Design review of the part shown in the three views and the two pictorial views. Dimensions are in mm from the part's minimum x, y and z. A direction names the side the tool comes from. Round coordinates to 2 decimals unless told otherwise and drop trailing zeros. Loops run counter-clockwise (first coordinate to the right, second up) from the corner with the lowest first, then second, coordinate; pieces in that order, holes last. Notation, with made-up numbers: M 6.25,13 L 61.25,13 A33 ccw 61.25,47 Z; hole C 62.25,75.5 d4. An arc over 180 degrees is marked long. Return JSON: item names as keys, results as strings. Group by question number.
Q1. Consider section C-C (z = 68). State the section outline as (x, y) points.
Q2. Clearance check with flat-ended pins moving along their axes: pin 1 Ø4 at (y, z) = (99, 36) entering from +X; pin 2 Ø11 at (x, z) = (128, 73.5) entering from +Y; pin 3 Ø1 at (x, z) = (59.5, 34.5) entering from +Y. State where each tip first meets the part, or that it passes through.
Q3. Consider section B-B (x = 67.5). State the section outline as (y, z) points, and give its area (3 significant figures).
Q4. For the marked faces 4, 5, 6 and 7, list the 3-axis set-ups (+Z, -Z, +X, -X, +Y, -Y) from which the entire face can be reached by the end or side of a thin tool; tool diameter is ignored.
Q5. Draft analysis for pull direction X (two halves, no side actions). For the marked faces 1, 2 and 3, state which applies: pulls with the +X half, pulls with the -X half, needs draft (parallel to the pull), parting line crosses it, or undercut.
Q6. Consider section A-A (y = 55). State the section outline as (x, z) points.
Q7. To check wall thickness, follow line 1 along X through (y, z) = (70.5, 10.5); line 2 along X through (y, z) = (42, 4.5); line 3 along Y through (x, z) = (14.5, 66.5). State the ranges of each line that lie inside material, in increasing order.
Q8. Consider section D-D (y = 97). State the section outline as (x, z) points, and give its area (3 significant figures).
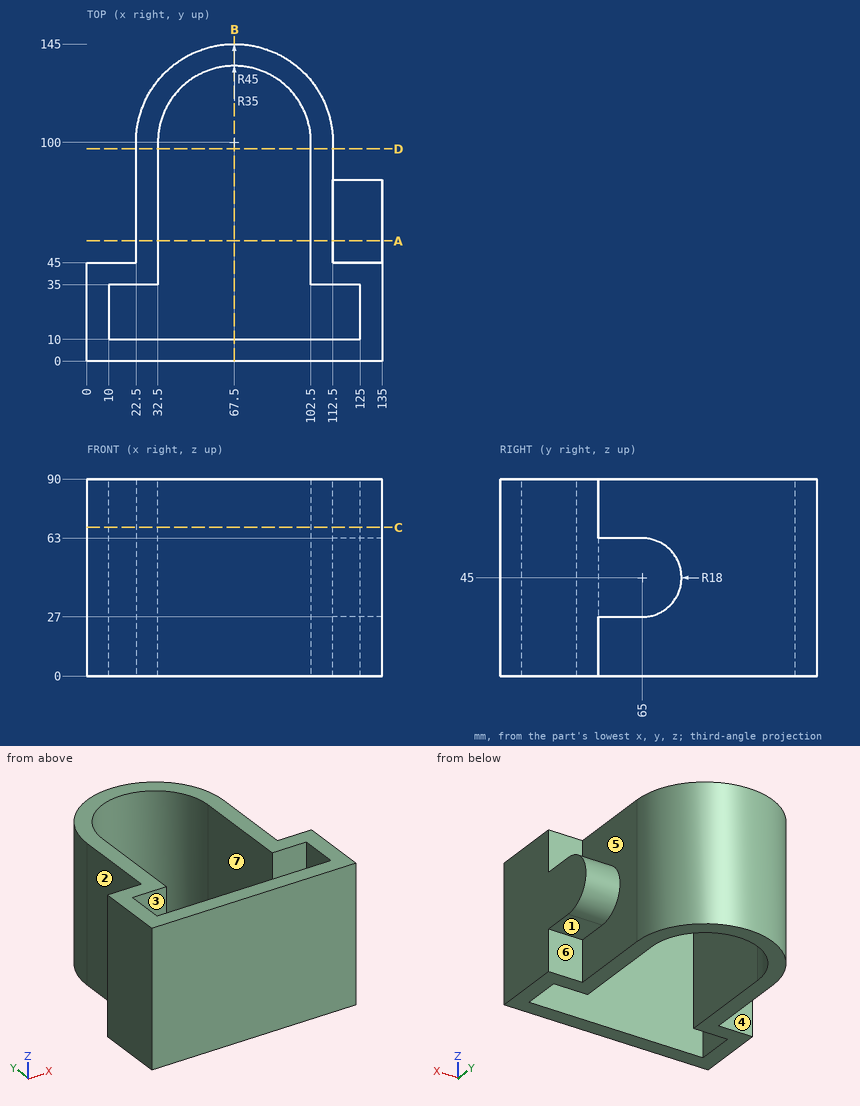
Values:
{
 "1": {"outline": "M 0,0 L 135,0 L 135,45 L 112.5,45 L 112.5,100 A45 ccw 22.5,100 L 22.5,45 L 0,45 Z; hole M 10,10 L 125,10 L 125,35 L 102.5,35 L 102.5,100 A35 ccw 32.5,100 L 32.5,35 L 10,35 Z"},
 "2": {"pin 1": "stops at x = 112.5", "pin 2": "stops at y = 45", "pin 3": "stops at y = 144.37"},
 "3": {"outline": "M 0,0 L 10,0 L 10,90 L 0,90 Z; M 135,0 L 145,0 L 145,90 L 135,90 Z", "area": "1,800 mm2"},
 "4": {"face 4": "+Z, -Z, -X, +Y", "face 5": "+X, +Y", "face 6": "-Z, +X, +Y", "face 7": "+Z, -Z"},
 "5": {"face 1": "needs draft", "face 2": "pulls with the -X half", "face 3": "undercut"},
 "6": {"outline": "M 22.5,0 L 32.5,0 L 32.5,90 L 22.5,90 Z; M 102.5,0 L 112.5,0 L 112.5,27 L 135,27 L 135,63 L 112.5,63 L 112.5,90 L 102.5,90 Z"},
 "7": {"line 1": "x = 22.5 to 32.5, 102.5 to 112.5", "line 2": "x = 0 to 32.5, 102.5 to 135", "line 3": "y = 0 to 10, 35 to 45"},
 "8": {"outline": "M 22.5,0 L 32.5,0 L 32.5,90 L 22.5,90 Z; M 102.5,0 L 112.5,0 L 112.5,90 L 102.5,90 Z", "area": "1,800 mm2"}
}
